The listing builds one solid part. Answer for the finished solid, in the listing's coordinates (mm). A direction names the side the tool comes from. Give positions to 0.01 mm unless a question says otherwise; leave off trailing zeros. Order: outer loops, then holes, each group sorted by start corner. A loop starts at its lowest first (then second) coordinate and runs counter-clockwise, first axis right, second up.
```python
from build123d import *

# Parameters (mm, degrees)
SKETCH1_W           = 26.5
SKETCH1_H           = 46.4
BOSS_EXTRUDE1_DEPTH = 8.75
SKETCH2_R           = 3.325
SKETCH2_R_2         = 1.27
BOSS_EXTRUDE2_DEPTH = 2.1
CUT_EXTRUDE1_DEPTH  = 0.127
FILLET1_R           = 1.27


with BuildPart() as part:
    # Sketch1 → Boss-Extrude1 (new, symmetric)
    with BuildSketch(Plane.XY):
        Rectangle(SKETCH1_W, SKETCH1_H)
    extrude(amount=BOSS_EXTRUDE1_DEPTH, both=True)

    # Sketch2 → Boss-Extrude2 (add)
    # profile 1 of 2: a face of its own
    with BuildSketch(Plane(origin=(0, 23.2, 0), x_dir=(1, 0, 0), z_dir=(0, 1, 0))):
        with Locations(Location((6.475, 0, 0), (0, 0, 90))):
            Circle(SKETCH2_R)
        with Locations(Location((6.475, 0, 0), (0, 0, 270))):
            Circle(SKETCH2_R_2, mode=Mode.SUBTRACT)
    # profile 2 of 2: a face of its own
    with BuildSketch(Plane(origin=(0, 23.2, 0), x_dir=(1, 0, 0), z_dir=(0, 1, 0))):
        Polygon((-6.475, 3.83937929), (-9.8, 1.919689645), (-9.8, -1.919689645), (-6.475, -3.83937929), (-3.15, -1.919689645), (-3.15, 1.919689645), align=None)
        with Locations(Location((-6.475, 0, 0), (0, 0, 270))):
            Circle(SKETCH2_R_2, mode=Mode.SUBTRACT)
    extrude(amount=BOSS_EXTRUDE2_DEPTH)

    # Sketch3 → Cut-Extrude1 (cut)
    # profile 1 of 2: a face of its own
    with BuildSketch(Plane.XY.offset(8.75)):
        with BuildLine():
            Line((-2.843132665, -0.135683761), (-3.222623183, 0.128263555))
            Line((-3.222623183, 0.128263555), (-1.751302403, 2.279063168))
            add(Edge.make_bspline(
                [(-1.751302403, 2.279063168), (-1.845177682, 2.267583179), (-2.03002334, 2.244978442), (-2.216194911, 2.240825761), (-2.307817828, 2.238782051)],
                knots=[0, 0, 0, 0, 1.015715272, 2, 2, 2, 2], degree=3))
            add(Edge.make_bspline(
                [(-2.307817828, 2.238782051), (-2.363368305, 2.240204869), (-2.472409033, 2.242997737), (-2.632718794, 2.265134756), (-2.786760058, 2.299228402), (-2.934124441, 2.350102115), (-3.075365836, 2.413327264), (-3.210175902, 2.49173013), (-3.338373165, 2.583965833), (-3.458580797, 2.689546665), (-3.567909259, 2.805476578), (-3.66531115, 2.928176181), (-3.746260242, 3.059070803), (-3.813504604, 3.195490302), (-3.864501837, 3.339395439), (-3.901638055, 3.489148699), (-3.924501614, 3.645799634), (-3.927221675, 3.752426915), (-3.92860275, 3.806565505)],
                knots=[0, 0, 0, 0, 1.060718605, 2.082097864, 3.085795603, 4.069760067, 5.054557537, 6.03741023, 7.043284206, 8.066802108, 9.088538119, 10.083643548, 11.053783639, 12.022749082, 12.983451788, 13.964007469, 14.966251758, 16, 16, 16, 16], degree=3))
            add(Edge.make_bspline(
                [(-3.92860275, 3.806565505), (-3.92598045, 3.880601444), (-3.920833407, 4.025918974), (-3.879409458, 4.238241458), (-3.811282517, 4.439002066), (-3.716291995, 4.627672954), (-3.596647832, 4.801540095), (-3.452852702, 4.958186445), (-3.285781232, 5.095384022), (-3.09923937, 5.213318758), (-2.897622303, 5.308168099), (-2.686456594, 5.378077517), (-2.467360245, 5.419199434), (-2.318940077, 5.424620914), (-2.244216065, 5.427350427)],
                knots=[0, 0, 0, 0, 1.022988612, 2.007919123, 2.978103895, 3.94594894, 4.918897164, 5.887013414, 6.875921846, 7.89917871, 8.930658928, 9.948724884, 10.967259574, 12, 12, 12, 12], degree=3))
            add(Edge.make_bspline(
                [(-2.244216065, 5.427350427), (-2.170906192, 5.424583395), (-2.026052794, 5.419116), (-1.813042034, 5.379074761), (-1.609024068, 5.311588363), (-1.415129862, 5.218327177), (-1.235607179, 5.101425329), (-1.074172322, 4.962126704), (-0.934509305, 4.800344538), (-0.816847009, 4.619991701), (-0.722398257, 4.426215432), (-0.654253258, 4.223946883), (-0.612304494, 4.014640721), (-0.607018381, 3.872832409), (-0.604350614, 3.801265358)],
                knots=[0, 0, 0, 0, 1.026385292, 2.028040595, 3.023318987, 4.028184125, 5.03290303, 6.015178782, 7.004435299, 8.016004309, 9.023023918, 10.015172535, 10.998308025, 12, 12, 12, 12], degree=3))
            add(Edge.make_bspline(
                [(-0.604350614, 3.801265358), (-0.606132256, 3.745712281), (-0.609745871, 3.633036762), (-0.635049573, 3.461843267), (-0.678018187, 3.287292003), (-0.726779683, 3.139546257), (-0.773848556, 3.017522768), (-0.818149077, 2.921136451), (-0.867304356, 2.819685731), (-0.924633918, 2.714234399), (-0.986262629, 2.603438185), (-1.055899868, 2.488408365), (-1.131957102, 2.368990578), (-1.186128226, 2.288486052), (-1.213867507, 2.247262286)],
                knots=[0, 0, 0, 0, 1.179839688, 2.393009684, 3.667231171, 4.993948276, 5.694988576, 6.444077775, 7.246288328, 8.089075292, 8.993003841, 9.939041771, 10.944649915, 12, 12, 12, 12], degree=3))
            Line((-1.213867507, 2.247262286), (-2.843132665, -0.135683761))
        make_face()
        with BuildLine():
            add(Edge.make_bspline(
                [(-2.219835389, 2.781517094), (-2.177753011, 2.782666722), (-2.095832926, 2.784904656), (-1.97582201, 2.798525772), (-1.86254375, 2.822676918), (-1.755695551, 2.85732934), (-1.654206069, 2.899143589), (-1.559687334, 2.952380758), (-1.472060244, 3.015905909), (-1.390738021, 3.087282956), (-1.318523403, 3.166583243), (-1.254202392, 3.24958244), (-1.199531058, 3.336644886), (-1.156346103, 3.42886089), (-1.120839662, 3.523985717), (-1.096319572, 3.62355123), (-1.082736116, 3.727038693), (-1.080420521, 3.797340236), (-1.079243776, 3.833066239)],
                knots=[0, 0, 0, 0, 1.163407946, 2.26475976, 3.333800367, 4.359385343, 5.366239384, 6.363380779, 7.350133999, 8.353570782, 9.349036268, 10.310270964, 11.253520213, 12.184142, 13.120487599, 14.056272588, 15.012232024, 16, 16, 16, 16], degree=3))
            add(Edge.make_bspline(
                [(-1.079243776, 3.833066239), (-1.080256252, 3.868807162), (-1.08225146, 3.939239033), (-1.098258449, 4.042879712), (-1.126418012, 4.142201665), (-1.164201245, 4.237748649), (-1.21397351, 4.32873564), (-1.273699018, 4.41630497), (-1.344656412, 4.499901401), (-1.426303149, 4.577558852), (-1.514348247, 4.649144366), (-1.608177813, 4.712320934), (-1.70701846, 4.765269647), (-1.810267177, 4.808962137), (-1.918139085, 4.843058274), (-2.030570353, 4.867577385), (-2.148129121, 4.881141824), (-2.227929399, 4.883442783), (-2.268596741, 4.884615385)],
                knots=[0, 0, 0, 0, 0.972161553, 1.915763587, 2.844109794, 3.775983486, 4.705125789, 5.659731448, 6.655561913, 7.682237399, 8.721216875, 9.739758359, 10.754845918, 11.767244016, 12.7857855, 13.828538656, 14.893392813, 16, 16, 16, 16], degree=3))
            add(Edge.make_bspline(
                [(-2.268596741, 4.884615385), (-2.308910401, 4.883440889), (-2.388005471, 4.881136539), (-2.50451914, 4.867603169), (-2.616190192, 4.842893377), (-2.723749546, 4.808977931), (-2.826995195, 4.765266388), (-2.92583118, 4.712318159), (-3.019682694, 4.649158909), (-3.107643379, 4.577502527), (-3.189434285, 4.500262871), (-3.259171692, 4.415938759), (-3.319033886, 4.328781192), (-3.368737759, 4.237736543), (-3.406539184, 4.142204896), (-3.434693877, 4.042878836), (-3.450702174, 3.939239261), (-3.452697203, 3.868807239), (-3.453709588, 3.833066239)],
                knots=[0, 0, 0, 0, 1.099389452, 2.15699305, 3.192601482, 4.213358962, 5.227959689, 6.245255729, 7.266013209, 8.307253147, 9.336162325, 10.327954924, 11.284637477, 12.215801273, 13.149702402, 14.080068371, 15.025723358, 16, 16, 16, 16], degree=3))
            add(Edge.make_bspline(
                [(-3.453709588, 3.833066239), (-3.452793485, 3.797312415), (-3.450986763, 3.72679933), (-3.433557843, 3.62319395), (-3.40441092, 3.523879657), (-3.365374461, 3.427890778), (-3.313967294, 3.336160707), (-3.25088481, 3.249124338), (-3.176944282, 3.165795027), (-3.093134128, 3.087467456), (-3.001409647, 3.015573096), (-2.903443138, 2.952783113), (-2.800921122, 2.899756918), (-2.693482704, 2.857209825), (-2.58192409, 2.823023144), (-2.465242642, 2.798570284), (-2.343824235, 2.785035309), (-2.261561524, 2.782701084), (-2.219835389, 2.781517094)],
                knots=[0, 0, 0, 0, 0.952633368, 1.87876736, 2.791047057, 3.707742249, 4.635551637, 5.587206343, 6.568248508, 7.601284464, 8.641511608, 9.671105535, 10.699146789, 11.713763218, 12.747829548, 13.806491675, 14.887386225, 16, 16, 16, 16], degree=3))
        make_face(mode=Mode.SUBTRACT)
    # profile 2 of 2: a face of its own
    with BuildSketch(Plane.XY.offset(8.75)):
        Polygon((0.14191007, 5.291666667), (0.650724173, 5.291666667), (2.413553032, 1.124691173), (4.177441921, 5.291666667), (4.687316053, 5.291666667), (2.448534002, 0), (2.380692122, 0), align=None)
    extrude(amount=-CUT_EXTRUDE1_DEPTH, mode=Mode.SUBTRACT)

    # Fillet1
    fillet1_edges = [part.edges().sort_by_distance(p)[0] for p in [
        (-13.25, 0, 8.75),
        (13.25, 0, 8.75),
        (-13.25, 0, -8.75),
        (13.25, 0, -8.75),
    ]]
    fillet(fillet1_edges, radius=FILLET1_R)


solid = part.part
```
1) Find section A-A (z = 0). Write down the section's boundary in (x, y) (3 decimals).
Geometry says:
outline: (-13.25, -23.2) - (13.25, -23.2) - (13.25, 23.2) - (9.8, 23.2) - (9.8, 25.3) - (7.745, 25.3) - (7.745, 23.2) - (5.205, 23.2) - (5.205, 25.3) - (3.15, 25.3) - (3.15, 23.2) - (-3.15, 23.2) - (-3.15, 25.3) - (-5.205, 25.3) - (-5.205, 23.2) - (-7.745, 23.2) - (-7.745, 25.3) - (-9.8, 25.3) - (-9.8, 23.2) - (-13.25, 23.2) - close
2) Find section C-C (z = 5.75). Write down the section's boundary in (x, y).
Geometry says:
outline: (-13.25, -23.2) - (13.25, -23.2) - (13.25, 23.2) - (-13.25, 23.2) - close
3) For a pull along X with two mould halves and no side action, classify faces 4 (the flat face through (-13.25, 0, 0)), 5 (the flat face through (6, 23.2, 0)), 6 (the cylindrical face through (-7.715, 24.235, -0.275)), 7 (the cylindrical face through (12.868, 0.325, -8.388)) as +X half, -X half, draft (parallel to the pull), parting line (faces both ways), or undercut.
Geometry says:
face 4: -X half
face 5: undercut
face 6: undercut
face 7: +X half
4) A tool of negligible diameter and unlimited length cuts with its end or side. For faces 1 (the cylindrical face through (9.72, 24.24, 0.72)), 2 (the flat face through (-4.789, 24.235, -2.866)), 3 (the flat face through (-8.161, 24.235, 2.866)), from which of +Z, -Z, +X, -X, +Y, -Y can it reach the whole face along a straight path? Write none if from no direction.
Geometry says:
face 1: +Y
face 2: -Z, +Y
face 3: +Z, -X, +Y
5) Given P1, Ø3.5, axis at x = -1.5, y = 2, coming from the +Z side; P2, Ø1.1, axis at y = 24.5, z = 0, coming from the +X side, each flat-ended and moving along its own axis, determine where each tip first touches the part or whether it passes through.
Geometry says:
P1: stops at z = 8.75
P2: stops at x = 9.8
6) Find section B-B (x = 11.25). Write down the section's boundary in (y, z), then the cut area to 3 significant figures.
Geometry says:
outline: (-23.2, -8.75) - (23.2, -8.75) - (23.2, 8.75) - (-23.2, 8.75) - close
area: 812 mm2
7) Straight lines are drawn through the part: probe 1 along X at (y, z) = (24.55, 0) (3 decimals); probe 2 along Y at (x, z) = (-0.25, 4.5). For each, find the intervals that lie inside material, in ascending order.
Geometry says:
probe 1: x = -9.8 to -7.745, -5.205 to -3.15, 3.15 to 5.205, 7.745 to 9.8
probe 2: y = -23.2 to 23.2
